Solid Edge part; units mm, degrees
sketch "Sketch1" plane through (0, 0, 0) normal (0, 0, 1) x (1, 0, 0)
  line L0 (-707.105, -705.605) -> (707.105, -705.605)
  line L1 (707.105, -705.605) -> (707.105, 705.605)
  line L2 (707.105, 705.605) -> (-707.105, 705.605)
  line L3 (-707.105, 705.605) -> (-707.105, -705.605)
extrude "Protrusion1" add sketch "Sketch1" against normal blind 18
sketch "Sketch2" plane through (0, 0, -18) normal (0, 0, -1) x (-1, 0, 0)
  circle A0 centre (-530.1407, 529.0161) radius 50
  circle A1 centre (530.1407, 529.0161) radius 50
  circle A2 centre (530.1407, -529.0161) radius 50
  circle A3 centre (-530.1407, -529.0161) radius 50
extrude "Kihúzás_2" add sketch "Sketch2" along normal blind 200
sketch "Sketch3" plane through (0, 0, 0) normal (0, 0, 1) x (0, -1, 0)
  circle A0 centre (0, 0) radius 10
extrude "Kivágás_1" cut sketch "Sketch3" along normal mid plane 923.1568
extrude "Kivágás_2" [suppressed]
The model under review builds one solid part; all positions refer to its coordinate system, in mm. A direction names the side the tool comes from. Give positions to 0.01 mm unless a question says otherwise; leave off trailing zeros. Write each loop counter-clockwise with the first axis right and the second up, starting at its lowest first coordinate (ties: lowest second). Pieces come first, ordered by that corner, then holes.
(1) Consider section A-A, the plane y = 425. Give the boundary of the cut face in (x, z) (3 decimals).
(2) To check wall thickness, follow L1, parallel to X at y = 0, z = -5 (3 decimals); L2, parallel to Z at x = 95.5, y = 273.5; L3, parallel to Y at x = 571, z = -57. State the ranges of each line that lie inside material, in increasing order.
(3) Consider section B-B, the plane x = 412. Give the boundary of the cut face in (y, z) (3 decimals), and give its area (3 significant figures).
(4) Tool access review of faces 1 (the cylindrical face through (482.45, -544.03, -116.6)), 2 (the flat face through (-529, -528, -218)): name each direction out of +Z, -Z, +X, -X, +Y, -Y from which nothing blocks a thin tool from reaching the whole face with its end or side.
(5) For P1, Ø10, axis at x = -39.5, y = -516, coming from the -Z side; P2, Ø6, axis at y = 517.5, z = -177, coming from the +X side; P3, Ø8, axis at x = -324, y = -21, coming from the +Z side, all flat-tipped, find the tip position at first contact; note any pin that passes through.
(6) The part is to be moulded in two halves that separate along X. For faces 3 (the cylindrical face through (-577.832, 513.997, -116.6)), 4 (the flat face through (531, 530, -218)), say which applies: released by +X, released by -X, zero draft, split by the parting line, or undercut.
(7) Consider section C-C, the plane z = -75.5. Give the boundary of the cut face in (x, y), and give its area (3 significant figures).
Returned:
1. outline: (-707.105, -18) - (707.105, -18) - (707.105, 0) - (-707.105, 0) - close
2. L1: x = -707.105 to -10, 10 to 707.105
2. L2: z = -18 to 0
2. L3: y = -557.83 to -500.2, 500.2 to 557.83
3. outline: (-705.605, -18) - (705.605, -18) - (705.605, 0) - (-705.605, 0) - close
3. area: 25,400 mm2
4. face 1: -Z
4. face 2: -Z, +X, -X, +Y, -Y
5. P1: stops at z = -18
5. P2: stops at x = 579.41
5. P3: stops at z = 0
6. face 3: undercut
6. face 4: zero draft
7. outline: circle Ø100 at (-530.14, -529.02); circle Ø100 at (-530.14, 529.02); circle Ø100 at (530.14, -529.02); circle Ø100 at (530.14, 529.02)
7. area: 31,400 mm2
